Input: dimensioned drawing with shaded views. Units: mm. Origin: part minimum x, y, z. A direction names the side the tool comes from. Round coordinates to 2 decimals unless told otherwise and drop trailing zeros. Loops run counter-clockwise (first coordinate to the right, second up) from the corner with the lowest first, then second, coordinate; pieces in that order, holes last. Notation, with made-up numbers: M 42.25,58 L 92.25,58 A28 ccw 92.25,89 Z; hole C 11.25,-31.5 d2. An arc over 180 degrees is marked long. Answer as CSV lines item,"result". Start each with the question number.
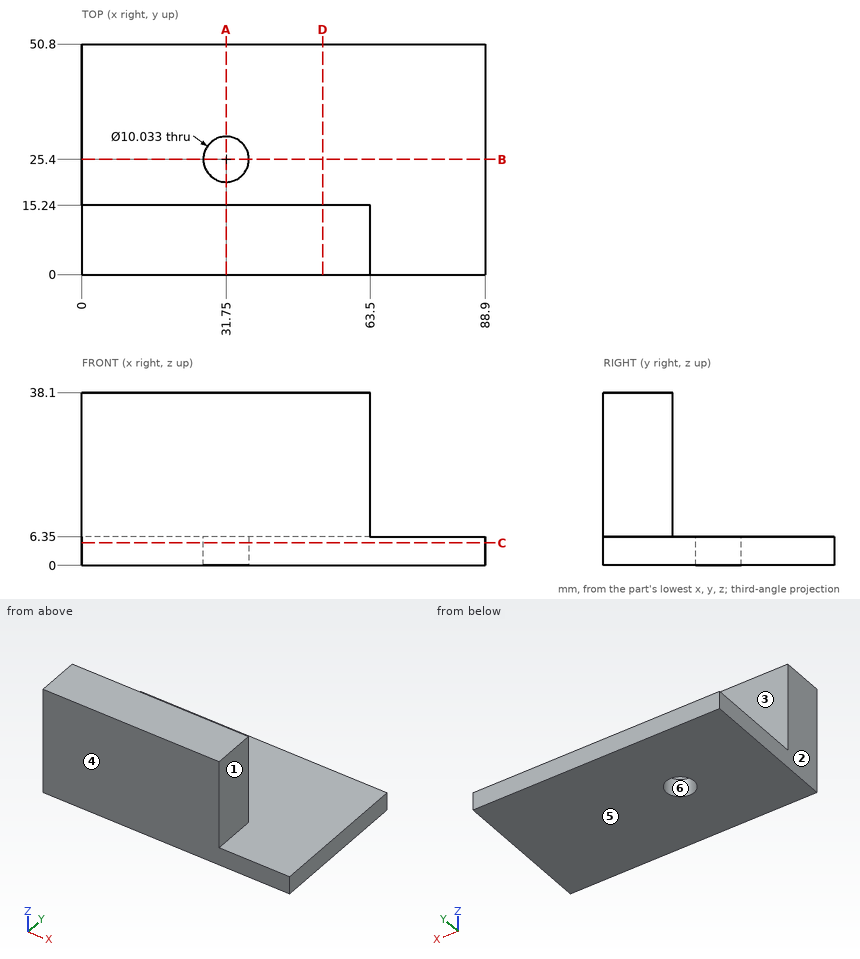
1) Ray query, line 1 along X through (y, z) = (25, 2); line 2 along Y through (x, z) = (31.75, 3.5); line 3 along Z through (x, y) = (13, 43). Return the intervals inside material, ascending.
2) Access query for the marked faces 1 and 2. Directions: +Z, -Z, +X, -X, +Y, -Y. A direction counts if a zero-diameter tool reaches every point of the face in a straight line with its end or side. Return the directions, or none.
3) Section A-A, the plane x = 31.75. Return loops of the section in (y, z).
4) Section D-D, the plane x = 53. Return loops of the section in (y, z), and give its area (3 significant figures).
5) Contact query for flat-ended pins moving along their axis: pin 1 Ø7.5 at (y, z) = (10, 29.5) entering from +X; pin 2 Ø9 at (x, y) = (31.75, 25.4) entering from -Z; pin 3 Ø4 at (x, y) = (35.5, 31) entering from +Z; pin 4 Ø9.5 at (x, z) = (26.5, 19) entering from +Y. Output: stop coordinate, or through.
6) Section C-C, the plane z = 5. Return loops of the section in (x, y).
7) Mould query, pull axis Y, two halves, no side actions, for the marked faces 3, 4, 5 and 6. Classes: pulls with the +Y half, pulls with the -Y half, needs draft (parallel to the pull), parting line crosses it, or undercut.
8) Section B-B, the plane y = 25.4. Return loops of the section in (x, z).
Findings below:
1,line 1,"0 to 26.75, 36.75 to 88.9"
1,line 2,"0 to 20.38, 30.42 to 50.8"
1,line 3,"0 to 6.35"
2,face 1,"+Z, +X, +Y, -Y"
2,face 2,"+Z, -Z, -X, +Y, -Y"
3,outline,"M 0,0 L 20.38,0 L 20.38,6.35 L 15.24,6.35 L 15.24,38.1 L 0,38.1 Z; M 30.42,0 L 50.8,0 L 50.8,6.35 L 30.42,6.35 Z"
4,outline,"M 0,0 L 50.8,0 L 50.8,6.35 L 15.24,6.35 L 15.24,38.1 L 0,38.1 Z"
4,area,"806 mm²"
5,pin 1,"x = 63.5"
5,pin 2,"through"
5,pin 3,"z = 6.35"
5,pin 4,"y = 15.24"
6,outline,"M 0,0 L 88.9,0 L 88.9,50.8 L 0,50.8 Z; hole C 31.75,25.4 d10.03"
7,face 3,"pulls with the +Y half"
7,face 4,"pulls with the -Y half"
7,face 5,"needs draft"
7,face 6,"undercut"
8,outline,"M 0,0 L 26.73,0 L 26.73,6.35 L 0,6.35 Z; M 36.77,0 L 88.9,0 L 88.9,6.35 L 36.77,6.35 Z"
